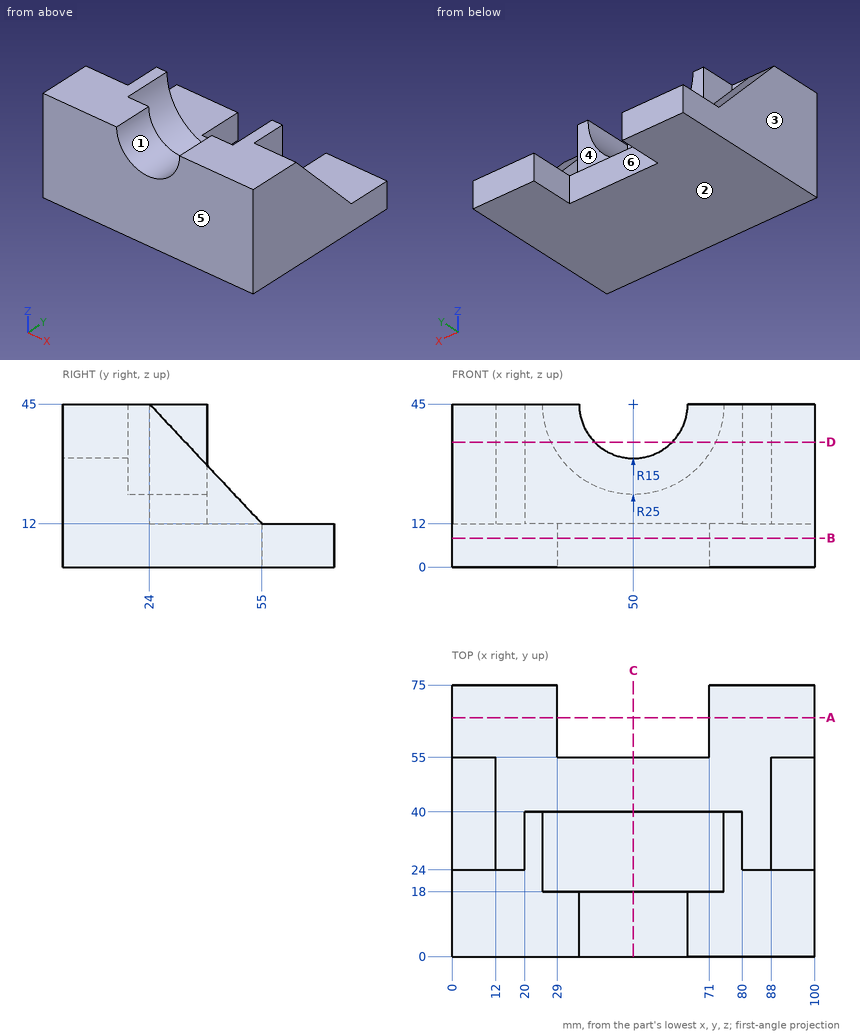
Could you check a few things on this drawing? It's one solid part, dimensions in mm from its lowest x, y, z. A direction names the side the tool comes from. Coordinates: 2 decimals unless noted, no trailing zeros. Loops run counter-clockwise (first coordinate to the right, second up) from the corner with the lowest first, then second, coordinate; pieces in that order, holes last. Notation, with made-up numbers: (38, 65.25) - (52, 65.25) arc R25 ccw to (52, 82.25) - close; hole circle Ø4 at (76.25, 30). An arc over 180 degrees is marked (long way). Return JSON: item names as keys, results as strings. Group by question number.
Item 1: If we section it at D-D on z = 34.5: Write out the boundary of the cut face in (x, y), and give its area (3 significant figures).
Item 2: I need wall thicknesses on line 1 (X direction, y = 32, z = 23); line 2 (Y direction, x = 37, z = 13); line 3 (Y direction, x = 68, z = 29). Which ranges of each line are inside material? Lowest first, please. Write a range as from..to.
Item 3: Will these pins go through, and if not, where does the flat tip stop? P1, Ø12, axis at x = 31, y = 66.5, coming from the +Z side; P2, Ø6.5, axis at x = 14.5, z = 22, coming from the +Y side; P3, Ø1.5, axis at x = 70, z = 28, coming from the +Y side.
Item 4: If we section it at C-C on x = 50: Write out the boundary of the cut face in (y, z), and give its area (3 significant figures).
Item 5: If we section it at A-A on y = 66: Write out the boundary of the cut face in (x, z).
Item 6: On a 3-axis mill with a long thin cutter (end or side, diameter ignored), from which of +Z, -Z, +X, -X, +Y, -Y can I reach the whole of each face in a straight line? I mean the marked faces 4, 5 and 6. Say none if no direction works.
Item 7: If we section it at B-B on z = 8: Write out the boundary of the cut face in (x, y), and give its area (3 significant figures).
Item 8: We'd pull the mould along X, two halves only. Please class the marked faces 1, 2 and 3: +X half, -X half, draft (parallel to the pull), parting line (faces both ways), or undercut.
Calculated:
{
 "1": {"outline": "(0, 0) - (39.29, 0) - (39.29, 18) - (27.31, 18) - (27.31, 40) - (20, 40) - (20, 24) - (12, 24) - (12, 33.86) - (0, 33.86) - close; (60.71, 0) - (100, 0) - (100, 33.86) - (88, 33.86) - (88, 24) - (80, 24) - (80, 40) - (72.69, 40) - (72.69, 18) - (60.71, 18) - close", "area": "2,210 mm^2"},
 "2": {"line 1": "x = 0..12, 20..38.13, 61.87..80, 88..100", "line 2": "y = 0..40", "line 3": "y = 0..18"},
 "3": {"P1": "stops at z = 12", "P2": "stops at y = 47.56", "P3": "stops at y = 40"},
 "4": {"outline": "(0, 0) - (55, 0) - (55, 12) - (40, 12) - (40, 20) - (18, 20) - (18, 30) - (0, 30) - close", "area": "1,160 mm^2"},
 "5": {"outline": "(0, 0) - (29, 0) - (29, 12) - (0, 12) - close; (71, 0) - (100, 0) - (100, 12) - (71, 12) - close"},
 "6": {"face 4": "+Z, +Y", "face 5": "+Z, -Z, +X, -X, -Y", "face 6": "+Z, -Z, +Y"},
 "7": {"outline": "(0, 0) - (100, 0) - (100, 75) - (71, 75) - (71, 55) - (29, 55) - (29, 75) - (0, 75) - close", "area": "6,660 mm^2"},
 "8": {"face 1": "undercut", "face 2": "draft", "face 3": "-X half"}
}
